Autodesk Inventor part; units mm, degrees
ref_plane "YZ Plane" through (0, 0, 0) normal (1, 0, 0) x (0, 1, 0)
ref_plane "XZ Plane" through (0, 0, 0) normal (0, 1, 0) x (-1, 0, 0)
ref_plane "XY Plane" through (0, 0, 0) normal (0, 0, 1) x (1, 0, 0)
sketch "Sketch1" plane through (0, 0, 0) normal (0, 1, 0) x (-1, 0, 0)
  line L0 (11.5, 6.25) -> (-11.5, 6.25)
  line L1 (-11.5, 6.25) -> (-11.5, -6.25)
  line L2 (-11.5, -6.25) -> (11.5, -6.25)
  line L3 (11.5, -6.25) -> (11.5, 6.25)
  line L4 (11.5, 6.25) -> (-11.5, -6.25) construction
  line L5 (-11.5, 6.25) -> (11.5, -6.25) construction
  line L6 (17, 8.5) -> (-17, 8.5)
  line L7 (-17, 8.5) -> (-17, -8.5)
  line L8 (-17, -8.5) -> (17, -8.5)
  line L9 (17, -8.5) -> (17, 8.5) construction
  line L10 (17, 8.5) -> (-17, -8.5) construction
  line L11 (-17, 8.5) -> (17, -8.5) construction
  line L12 (38.8, 0) -> (-26.3, 0)
  line L13 (0, -20.3) -> (0, 20.3)
  line L14 (29.5, 14.5) -> (18.5, 14.5)
  line L15 (18.5, 14.5) -> (18.5, -14.5) construction
  line L16 (18.5, -14.5) -> (29.5, -14.5)
  line L17 (29.5, -14.5) -> (29.5, 14.5)
  line L18 (29.5, 14.5) -> (18.5, -14.5) construction
  line L19 (18.5, 14.5) -> (29.5, -14.5) construction
  line L20 (18.5, 14.5) -> (17, 8.5)
  line L21 (17, -8.5) -> (18.5, -14.5)
  circle A0 centre (-14, 0) radius 1.15
  circle A1 centre (14, 0) radius 1.15
  circle A2 centre (24, 9.25) radius 1.25
  circle A3 centre (24, -9.25) radius 1.25
  point P0 (0, 0)
  point P1 (24, 0)
  dimension "d0" = 23
  dimension "d1" = 12.5
  dimension "d2" = 17
  dimension "d3" = 34
  dimension "d11" = 2.3
  dimension "d12" = 28
  dimension "d13" = 12.5
  dimension "d14" = 2.5
  dimension "d15" = 9.25
  dimension "d16" = 29
  dimension "d18" = 5.5
extrude "Extrusion1" add sketch "Sketch1" along normal blind 4 contours L0 L13 L6 L20 L14 L17 L12 A1 L3 | L0 L1 L12 A0 L7 L6 L13 | L12 A1 L17 L16 L21 L8 L13 L2 L3 | L1 L2 L13 L8 L7 L12 A0
sketch "Sketch2" plane through (0, 4, 0) normal (0, 1, 0) x (1, 0, 0)
  circle A0 centre (14, 0) radius 1.15
  circle A1 centre (14, 0) radius 2
  line L0 (0, 20.3) -> (0, -20.3)
  circle A2 centre (-14, 0) radius 2
  point P0 (0, 0)
  dimension "d21" = 4
extrude "Extrusion2" cut sketch "Sketch2" against normal blind 2
sketch "Sketch3" plane through (0, 0, 0) normal (0, -1, 0) x (1, 0, 0)
  line L0 (-38.8, 0) -> (26.3, 0)
  circle A0 centre (-24, 9.25) radius 1.25
  circle A1 centre (-24, 9.25) radius 2.25
  circle A2 centre (-24, -9.25) radius 2.25
  point P0 (0, 0)
  dimension "d24" = 4.5
extrude "Extrusion3" cut sketch "Sketch3" against normal blind 2 contours A0 | A1 | A2
fillet "Fillet1" radius 5 8 edges at (-18.5, 2, 14.5) (-17, 2, 8.5) (-29.5, 2, 14.5) (-29.5, 2, -14.5) (-18.5, 2, -14.5) (-17, 2, -8.5) (17, 2, -8.5) (17, 2, 8.5)
properties part number "mount1"
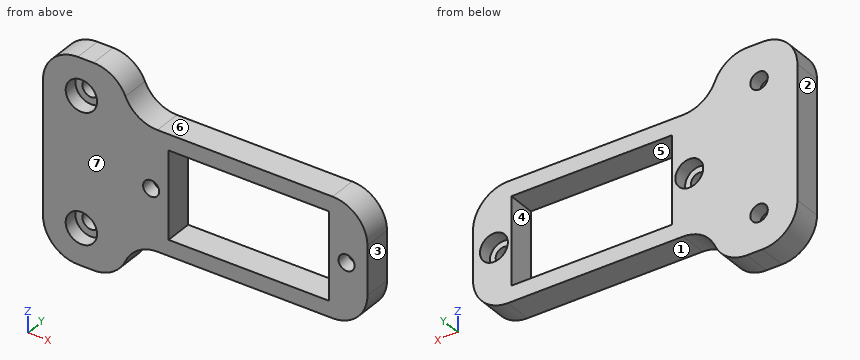
Verification items for the finished model (mm, model axes). Face numbers are marked on the shaded views. A direction names the side the tool comes from. Give positions to 0.01 mm unless a question says otherwise; leave off trailing zeros. Order: outer loops, then holes, each group sorted by start corner. A loop starts at its lowest first (then second) coordinate and runs counter-clockwise, first axis right, second up. Notation, with made-up numbers: M 3,44 L 8,44 A22 cw 8,57 Z; hole C -5.75,37.25 d7. An arc over 180 degrees is marked long. Answer in a Markdown table with one row per item. Add a question column.
Item 1: Section check B-B, the plane z = 0. Enter the section's corners in (x, y), and give its area (3 significant figures).
Item 2: Section check D-D, the plane x = -23.5. Enter the section's corners in (y, z), and give its area (3 significant figures).
Item 3: Scan lines: probe 1 along Z at (x, y) = (-24, 0.9); probe 2 along Z at (x, y) = (-24, 3.25); probe 3 along Z at (x, y) = (-1, 1.25). Record each from-to range of solid material in increasing order. Write a range as from..to.
Item 4: Mould release check, pull along X, two halves, no side actions. Record for the marked faces 1, 2, 3 and 4: released by +X, released by -X, zero draft, split by the parting line, or undercut.
Item 5: Tool access check on the marked faces 5, 6 and 7. Record the directions out of +Z, -Z, +X, -X, +Y, -Y that give a thin tool (end or side, any length) a straight path to the whole face; none if there is none.
Item 6: Section check C-C, the plane y = 1.55. State how many separate pieces and enclosed holes the cut face has, and give its area (3 significant figures).
Item 7: Section check A-A, the plane x = 9. Enter the section's corners in (y, z).
Item 8: Gauge pin test, flat ends, axial feed: pin 1 (3.5 mm diameter, centred on x = -23.5, z = 9.5, fed in from -Y); pin 2 (3 mm diameter, centred on x = -14, z = 0, fed in from +Y); pin 3 (2 mm diameter, centred on x = -4.5, y = 1.5, fed in from +Z); pin 4 (1.2 mm diameter, centred on x = 1.5, y = 1.5, fed in from -Z). Record the tip position at first contact, or that the pin passes through.
Filled sheet:
| question | item | result |
|---|---|---|
| 1 | outline | M -29.5,0 L -15.15,0 L -15.15,2 L -16,2 L -16,4 L -29.5,4 Z; M -12.85,0 L -11.5,0 L -11.5,4 L -12,4 L -12,2 L -12.85,2 Z; M 11.5,0 L 12.85,0 L 12.85,2 L 12,2 L 12,4 L 11.5,4 Z; M 15.15,0 L 17,0 L 17,4 L 16,4 L 16,2 L 15.15,2 Z |
| 1 | area | 68.8 mm^2 |
| 2 | outline | M 0,-14.5 L 4,-14.5 L 4,-10.4 L 2,-10.4 L 2,-11.44 L 0,-11.44 Z; M 0,-7.06 L 2,-7.06 L 2,-8.1 L 4,-8.1 L 4,8.1 L 2,8.1 L 2,7.06 L 0,7.06 Z; M 0,11.44 L 2,11.44 L 2,10.4 L 4,10.4 L 4,14.5 L 0,14.5 Z |
| 2 | area | 89.3 mm^2 |
| 3 | probe 1 | z = -14.5..-11.5, -7..7, 11.5..14.5 |
| 3 | probe 2 | z = -14.5..-10.5, -8..8, 10.5..14.5 |
| 3 | probe 3 | z = -8.5..-6.25, 6.25..8.5 |
| 4 | face 1 | zero draft |
| 4 | face 2 | released by -X |
| 4 | face 3 | released by +X |
| 4 | face 4 | undercut |
| 5 | face 5 | +Y, -Y |
| 5 | face 6 | +Z, +X, +Y, -Y |
| 5 | face 7 | +Z, -Z, +X, -X, -Y |
| 6 | separate pieces | 1 |
| 6 | enclosed holes | 5 |
| 6 | area | 583 mm^2 |
| 7 | outline | M 0,-8.5 L 4,-8.5 L 4,-6.25 L 0,-6.25 Z; M 0,6.25 L 4,6.25 L 4,8.5 L 0,8.5 Z |
| 8 | pin 1 | stops at y = 0 |
| 8 | pin 2 | stops at y = 2 |
| 8 | pin 3 | stops at z = 8.5 |
| 8 | pin 4 | stops at z = -8.5 |
